Input: part model. Units: mm. Frame: model coordinates. Give positions to 0.01 mm unless a question says otherwise; leave off trailing zeros. Loops run counter-clockwise (first coordinate to the right, second up) from the corner with the lowest first, then second, coordinate; pieces in that order, holes last. Notation, with made-up numbers: M 62,15.5 L 109,15.5 A26 ccw 109,54.5 Z; hole C 9,-34.5 d3. An arc over 180 degrees is marked long. Use CSV: the item, a comma, the result in double quotes. Start each with the question number.
Q1. Section A-A, the plane z = 37.5. Output: boundary loops of the cut face in (x, y), plus the area to 3 significant figures.
Q2. Section B-B, the plane z = 29. Output: boundary loops of the cut face in (x, y).
Q3. Pin query (flat end, axial travel): pin 1 (10 mm diameter, centred on y = -11, z = 14, fed in from +X); pin 2 (12 mm diameter, centred on x = 0, y = 0, fed in from +Z); pin 3 (10 mm diameter, centred on x = 2.5, y = -14.5, fed in from -Z); pin 4 (5 mm diameter, centred on x = -6, z = 14.5, fed in from -Y). Return the tip coordinate at first contact, or that it passes through.
Q4. Material intervals for line 1 along Y through (x, z) = (0, 3.75); line 2 along Y through (x, z) = (3, 37); line 3 along X through (y, z) = (1.5, 38), sorted ascending.
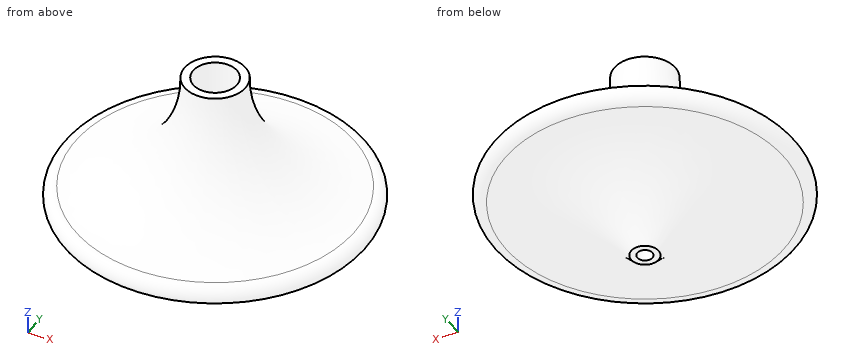
from build123d import *


# Not quite as in the source:
# - a feature names something its author has since deleted; it is built from what else it names


with BuildPart() as f1:
    # F0 (on Front) → F1 (revolve)
    with BuildSketch(Plane.XZ):
        with BuildLine():
            Line((1.579833799, 13.9581533149), (1.579833799, 0))
            Line((1.579833799, 0), (2.8451390099, 0))
            ThreePointArc((2.8451390099, 0), (14.581897199, 8.8414692128), (28.9212949574, 12.0515692979))
            ThreePointArc((28.9212949574, 12.0515692979), (31.4253055765, 13.9538953081), (28.9212949574, 15.8562213182))
            ThreePointArc((28.9212949574, 15.8562213182), (12.6572464777, 23.8517040301), (6.334674079, 40.8361703157))
            Line((6.334674079, 40.8361703157), (4.5473091304, 40.8361703157))
            Line((4.5473091304, 40.8361703157), (4.5473091304, 31.7337363958))
            Line((4.5473091304, 31.7337363958), (0, 31.7337363958))
            Line((0, 31.7337363958), (0, 13.9581533149))
            Line((0, 13.9581533149), (1.579833799, 13.9581533149))
        make_face()
    revolve(axis=Axis((0, 0, 22.8459448554), (0, 0, 1)))


solid = f1.part
A:
1,outline,"C 0,0 d12.98; hole C 0,0 d9.09"
1,area,"67.3 mm^2"
2,outline,"C 0,0 d18.17"
3,pin 1,"x = 30.85"
3,pin 2,"z = 40.84"
3,pin 3,"z = 6.1"
3,pin 4,"y = -31.22"
4,line 1,"-6.62 to -1.58, 1.58 to 6.62"
4,line 2,"-5.82 to -3.42, 3.42 to 5.82"
4,line 3,"-6.26 to -4.29, 4.29 to 6.26"
